```python
from build123d import *

# Parameters (mm, degrees)
F1_DEPTH = 4.5
F2_R     = 1.5
F3_DEPTH = 20.001
F4_R     = 4


with BuildPart() as f1:
    # F0 (on Top) → F1 (new body, symmetric)
    with BuildSketch(Plane.XY):
        Polygon((-5, 25), (-10, 25), (-10, 0), (-4.5, 0), (-4.5, -25), (4.5, -25), (4.5, 0), (10, 0), (10, 25), (5, 25), (5, 14), (-5, 14), align=None)
    extrude(amount=F1_DEPTH, both=True)

    # F2 (on face) → F3 (cut, through all)
    with BuildSketch(Plane.YZ.offset(10)):
        with Locations((20, 0)):
            Circle(F2_R)
        with Locations((-20, 0)):
            Circle(F2_R)
    extrude(amount=-F3_DEPTH, mode=Mode.SUBTRACT)

    # F4
    f4_edges = [f1.edges().sort_by_distance(p)[0] for p in [
        (-7.5, 25, 4.5),
        (10, 0, 0),
        (-10, 0, 0),
        (0, -25, 4.5),
        (0, -25, -4.5),
        (-7.5, 25, -4.5),
        (7.5, 25, -4.5),
        (7.5, 25, 4.5),
    ]]
    fillet(f4_edges, radius=F4_R)


solid = f1.part
```
Design review of the part built by this model. Coordinates are the model's own, in mm. A direction names the side the tool comes from. Give positions to 0.01 mm unless a question says otherwise; leave off trailing zeros. Order: outer loops, then holes, each group sorted by start corner. A loop starts at its lowest first (then second) coordinate and runs counter-clockwise, first axis right, second up. Notation, with made-up numbers: (8, 58) - (46, 58) arc R18 cw to (46, 88) - close; hole circle Ø2 at (71.25, 13.25). An arc over 180 degrees is marked (long way). Use a Markdown table: item, result. Add a question column.
(1) Add section B-B on x = -5.5. Give the boundary of the cut face in (y, z), then the cut area to 3 significant figures.
(2) Machinability: for faces 4 (the face through (-4.5, -12, 0)), 5 (the face through (4.5, -13, 0)), 6 (the face through (5, 18, 0)), which of the approach directions +Z, -Z, +X, -X, +Y, -Y give a long, thin tool a straight path to every point of the face, cutting with its end or side? Answer none if there is none.
(3) Wall thickness on probe 1 along X at (y, z) = (20.5, 3.5); probe 2 along Z at (x, y) = (-7.8, 20); probe 3 along X at (y, z) = (-15, 1.5): over which ranges is each line inside the solid? List them lowest first. Write a range as [from, to].
(4) Add section A-A on y = -20. Give the boundary of the cut face in (x, z), then the cut area to 3 significant figures.
(5) Clearance check with flat-ended pins moving along their axes: P1, Ø4.5, axis at y = -11.5, z = 2, coming from the +X side; P2, Ø4, axis at y = -20, z = 0, coming from the -X side; P3, Ø0.5, axis at x = 5, z = -0.5, coming from the -Y side. State where each tip first meets the part, or that it passes through.
(6) Add section C-C on z = 0. Give the boundary of the cut face in (x, y).
(7) Mouldability with a two-part tool opening along Z and no side actions: class faces 1 (the face through (0.06, -21.5, 0.07)), 2 (the face through (0, 0, 4.5)), 3 (the face through (10, 14, 0)) as +Z half, -Z half, draft (parallel to the pull), parting line (faces both ways), or undercut.
(8) Add section D-D on y = 20. Give the boundary of the cut face in (x, z).
Report:
| question | item | result |
|---|---|---|
| 1 | outline | (0, -4.5) - (21, -4.5) arc R4 ccw to (25, -0.5) - (25, 0.5) arc R4 ccw to (21, 4.5) - (0, 4.5) - close; hole circle Ø3 at (20, 0) |
| 1 | area | 211 mm² |
| 2 | face 4 | +Z, -Z, -X, -Y |
| 2 | face 5 | +Z, -Z, +X, -Y |
| 2 | face 6 | +Z, -Z, +Y |
| 3 | probe 1 | x = [-10, -5], [5, 10] |
| 3 | probe 2 | z = [-4.5, -1.5], [1.5, 4.5] |
| 3 | probe 3 | x = [-4.5, 4.5] |
| 4 | outline | (-4.5, -4.5) - (4.5, -4.5) - (4.5, -1.5) - (-4.5, -1.5) - close; (-4.5, 1.5) - (4.5, 1.5) - (4.5, 4.5) - (-4.5, 4.5) - close |
| 4 | area | 54.0 mm² |
| 5 | P1 | stops at x = 4.5 |
| 5 | P2 | stops at x = -4.5 |
| 5 | P3 | stops at y = 0 |
| 6 | outline | (-10, 4) arc R4 ccw to (-6, 0) - (-4.5, 0) - (-4.5, -18.5) - (4.5, -18.5) - (4.5, 0) - (6, 0) arc R4 ccw to (10, 4) - (10, 18.5) - (5, 18.5) - (5, 14) - (-5, 14) - (-5, 18.5) - (-10, 18.5) - close; (-10, 21.5) - (-5, 21.5) - (-5, 25) - (-10, 25) - close; (-4.5, -25) - (4.5, -25) - (4.5, -21.5) - (-4.5, -21.5) - close; (5, 21.5) - (10, 21.5) - (10, 25) - (5, 25) - close |
| 7 | face 1 | undercut |
| 7 | face 2 | +Z half |
| 7 | face 3 | draft |
| 8 | outline | (-10, -4.5) - (-5, -4.5) - (-5, -1.5) - (-10, -1.5) - close; (-10, 1.5) - (-5, 1.5) - (-5, 4.5) - (-10, 4.5) - close; (5, -4.5) - (10, -4.5) - (10, -1.5) - (5, -1.5) - close; (5, 1.5) - (10, 1.5) - (10, 4.5) - (5, 4.5) - close |
